from build123d import *

# Parameters (mm, degrees)
SKETCH1_R                         = 260
BOSS_EXTRUDE1_DEPTH               = 20
SKETCH2_R                         = 100
CUT_EXTRUDE1_DEPTH                = 20
F_1_2_13_TAPPED_HOLE1_D           = 10.71626
F_1_2_13_TAPPED_HOLE1_DEPTH       = 70.4
F_1_2_13_TAPPED_HOLE1_CBORE_D     = 12.7
F_1_2_13_TAPPED_HOLE1_CBORE_DEPTH = 64.5
F_1_2_13_TAPPED_HOLE1_TIP         = 3.219489309


with BuildPart() as part:
    # Sketch1 → Boss-Extrude1 (new body)
    with BuildSketch(Plane(origin=(0, 0, 0), x_dir=(0, 0, -1), z_dir=(1, 0, 0))):
        Circle(SKETCH1_R)
    extrude(amount=BOSS_EXTRUDE1_DEPTH)

    # Sketch2 → Cut-Extrude1 (cut)
    with BuildSketch(Plane(origin=(20, 0, 0), x_dir=(0, 0, -1), z_dir=(1, 0, 0))):
        Circle(SKETCH2_R)
    extrude(amount=-CUT_EXTRUDE1_DEPTH, mode=Mode.SUBTRACT)

    # 1/2-13 Tapped Hole1
    with Locations(Plane(origin=(20, 176.776695297, -177.367627121), x_dir=(0, 0, 1), z_dir=(1, 0, 0))):
        with Locations((0, 0), (354.144322418, 0), (177.367627121, 426.776695297), (177.367627121, 316.776695297)):
            CounterBoreHole(F_1_2_13_TAPPED_HOLE1_D / 2, F_1_2_13_TAPPED_HOLE1_CBORE_D / 2, F_1_2_13_TAPPED_HOLE1_CBORE_DEPTH, depth=F_1_2_13_TAPPED_HOLE1_DEPTH)
            with Locations((0, 0, -(F_1_2_13_TAPPED_HOLE1_DEPTH + F_1_2_13_TAPPED_HOLE1_TIP / 2))):  # 118° drill point
                Cone(0, F_1_2_13_TAPPED_HOLE1_D / 2, F_1_2_13_TAPPED_HOLE1_TIP, mode=Mode.SUBTRACT)


solid = part.part
Can you work these out from the model? Positions are in its coordinate system, mm. Coordinates: 2 decimals unless noted, no trailing zeros. Loops run counter-clockwise (first coordinate to the right, second up) from the corner with the lowest first, then second, coordinate; pieces in that order, holes last. Notation, with made-up numbers: (-21.75, 64.5) - (0.25, 64.5) arc R22 cw to (0.25, 98.5) - close; hole circle Ø7 at (57, 26.25). An arc over 180 degrees is marked (long way). Answer as a JSON object with one key per item and string values. Group by question number.
Item 1: If we section it at A-A (y = 0): List the corners of the cut face in (x, z) for me, plus the area to 3 significant figures.
Item 2: If I drill on L1, parallel to Y at x = 13.5, z = 0; L2, parallel to Z at x = 18, y = -57.5; L3, parallel to Z at x = 12, y = 84, over which ranges is the centre line in solid material (lowest first)? Write a range as from..to.
Item 3: For pin 1 (10 mm diameter, centred on y = 176.78, z = -177.37, fed in from +X); pin 2 (6 mm diameter, centred on x = 7.5, y = 30.5, fed in from -Z); pin 3 (6 mm diameter, centred on x = 3.5, y = -51.5, fed in from +Z); pin 4 (2 mm diameter, centred on x = 3, z = -92, fed in from +Y), each with a flat end and sliding along its axis, tell me the tip position at first contact or that it passes through.
Item 4: If we mould it in two halves opening along Z, with no side actions, what happens to faces 1 (the face through (10.14, 30.04, -95.38)), 2 (the face through (9.86, 78.097, -247.994)), 3 (the face through (0, 4, -112))? For each: released by +Z, released by -Z, zero draft, split by the parting line, or undercut.
Item 5: If we section it at C-C (y = -140): List the corners of the cut face in (x, z) for me.
Item 6: If we section it at B-B (x = 6.5): List the corners of the cut face in (y, z) for me, plus the area to 3 significant figures.
Item 7: If we section it at D-D (z = -198.5): List the corners of the cut face in (x, y) for me, plus the area to 3 significant figures.
Returned:
{
 "1": {"outline": "(0, -260) - (20, -260) - (20, -100) - (0, -100) - close; (0, 100) - (20, 100) - (20, 260) - (0, 260) - close", "area": "6,400 mm²"},
 "2": {"L1": "y = -260..-256.35, -243.65..-146.35, -133.65..-100, 100..260", "L2": "z = -253.56..-81.82, 81.82..253.56", "L3": "z = -246.06..-54.26, 54.26..246.06"},
 "3": {"pin 1": "passes through", "pin 2": "stops at z = -258.54", "pin 3": "stops at z = 255.44", "pin 4": "stops at y = 243.55"},
 "4": {"face 1": "undercut", "face 2": "split by the parting line", "face 3": "zero draft"},
 "5": {"outline": "(0, -219.09) - (20, -219.09) - (20, -6.35) - (0, -6.35) - close; (0, 6.35) - (20, 6.35) - (20, 219.09) - (0, 219.09) - close"},
 "6": {"outline": "circle Ø520 at (0, 0); hole circle Ø12.7 at (-250, 0); hole circle Ø12.7 at (-140, 0); hole circle Ø200 at (0, 0); hole circle Ø12.7 at (176.78, -177.37); hole circle Ø12.7 at (176.78, 176.78)", "area": "180,000 mm²"},
 "7": {"outline": "(0, -167.92) - (20, -167.92) - (20, 167.92) - (0, 167.92) - close", "area": "6,720 mm²"}
}
